Geometry: final body of the model. Coordinates: model frame, mm. A direction names the side the tool comes from. Coordinates: 2 decimals unless noted, no trailing zeros. Loops run counter-clockwise (first coordinate to the right, second up) from the corner with the lowest first, then second, coordinate; pieces in that order, holes last. Notation, with made-up numbers: (88.25, -18.5) -> (116.25, -18.5) arc R30 cw to (116.25, 12.5) -> close; hole circle Ø8 at (25.5, -28.75). An arc over 180 degrees is marked (long way). One line per item, written item: value. Start each with the question number.
Item 1: Mould query, pull axis Y, two halves, no side actions, for faces 4 (the flat face through (19.05, 13, -3)), 5 (the flat face through (20.5, 27, -2)), 6 (the cylindrical face through (9.27, 2.54, -14.83)). Classes: +Y half, -Y half, draft (parallel to the pull), parting line (faces both ways), or undercut.
Item 2: Section query A-A on z = -4. Return loops of the section in (x, y), then the cut area to 3 significant figures.
Item 3: Set-up query: faces 1 (the flat face through (12, 27, -1)), 2 (the flat face through (13, 15, -9.3)), 3 (the flat face through (5.7, 8.8, -4.8)). Return all of +Z, -Z, +X, -X, +Y, -Y with unobstructed straight access to the full face (end or side cutting, diameter ignored); none if empty.
Item 4: Ray query, probe 1 along Y at (x, z) = (23, -0.45); probe 2 along Y at (x, z) = (11, -1.5); probe 3 along Z at (x, y) = (18.75, 12). Return the intervals inside material, ascending. Write a range as from..to.
Item 5: Section query B-B on x = 15.5. Return loops of the section in (y, z).
Item 6: Contact query for flat-ended pins moving along their axis: pin 1 Ø5.5 at (x, y) = (9, 29) entering from +Z; pin 2 Ø12 at (x, y) = (14.5, 26) entering from -Z; pin 3 Ø1.1 at (y, z) = (13.5, -2.5) entering from +X; pin 4 Ø8 at (y, z) = (23.5, -7.5) entering from +X. Output: stop coordinate, or through.
Item 7: Section query C-C on y = 24.5. Return loops of the section in (x, z).
Item 8: Section query D-D on y = 8. Return loops of the section in (x, z), then the cut area to 3 significant figures.
from build123d import *

# Parameters (mm, degrees)
SKETCH_1_W             = 25
SKETCH_1_H             = 24
EXTRUDE_354_DEPTH      = 1
EXTRUDE_536_DEPTH      = 3.8
SKETCH_3_W             = 22
SKETCH_3_H             = 4.802295703
EXTRUDE_803_DEPTH      = 1.5
HOLE_WIZARD_953_D      = 0.5
HOLE_WIZARD_953_DEPTH  = 1
HOLE_WIZARD_1615_D     = 2
HOLE_WIZARD_1615_DEPTH = 16.4
SKETCH_12_W            = 16
SKETCH_12_H            = 1.5
EXTRUDE_2779_DEPTH     = 7.5


with BuildPart() as part:
    # Эскиз1 → Extrude 354 (new body)
    with BuildSketch(Plane(origin=(0, 0, -1), x_dir=(-1, 0, 0), z_dir=(0, 0, -1))):
        with Locations((-12.5, 12)):
            Rectangle(SKETCH_1_W, SKETCH_1_H)
    extrude(amount=-EXTRUDE_354_DEPTH)

    # Эскиз2 → Extrude 536 (add)
    with BuildSketch(Plane(origin=(0, 0, -1), x_dir=(-1, 0, 0), z_dir=(0, 0, -1))):
        with BuildLine():
            Line((-5.95, 10.75), (-3.949995117, 10.75))
            ThreePointArc((-3.949995117, 10.75), (-1.949995117, 8.75), (-3.949995117, 6.75))
            Line((-3.949995117, 6.75), (-5.95, 6.75))
            Line((-5.95, 6.75), (-5.95, 2.2))
            Line((-5.95, 2.2), (-19.05, 2.2))
            Line((-19.05, 2.2), (-19.05, 6.75))
            Line((-19.05, 6.75), (-21.050009766, 6.75))
            ThreePointArc((-21.050009766, 6.75), (-23.050009766, 8.75), (-21.050009766, 10.75))
            Line((-21.050009766, 10.75), (-19.05, 10.75))
            Line((-19.05, 10.75), (-19.05, 15.3))
            Line((-19.05, 15.3), (-5.95, 15.3))
            Line((-5.95, 15.3), (-5.95, 10.75))
        make_face()
    extrude(amount=EXTRUDE_536_DEPTH)

    # Эскиз3 → Extrude 803 (add)
    with BuildSketch(Plane(origin=(0, 0, -1), x_dir=(-1, 0, 0), z_dir=(0, 0, -1))):
        with Locations((-12.5, 21.098852149)):
            Rectangle(SKETCH_3_W, SKETCH_3_H)
    extrude(amount=EXTRUDE_803_DEPTH)

    # Эскиз4 → Revolve 894 (revolve)
    with BuildSketch(Plane.XZ.offset(-8.75), mode=Mode.PRIVATE) as revolve_894_sk:
        Polygon((19.1, -4.8), (12.5, -4.8), (12.5, -16.4), (19.5, -16.4), (19.5, -13.3), (18.25, -13.3), (18.25, -9.3), (19.1, -9.3), align=None)
    revolve(revolve_894_sk.sketch.rotate(Axis((12.5, 8.75, -4.8), (0, 0, -1)), 180), axis=Axis((12.5, 8.75, -4.8), (0, 0, -1)))

    # Hole Wizard 953
    with Locations(Plane.XY):
        with Locations((12.5, 8.75)):
            Hole(HOLE_WIZARD_953_D / 2, depth=HOLE_WIZARD_953_DEPTH)

    # Hole Wizard 1615
    with Locations(Plane.XY):
        with Locations((2, 2), (2, 15.5), (23, 15.5), (23, 2)):
            Hole(HOLE_WIZARD_1615_D / 2, depth=HOLE_WIZARD_1615_DEPTH)

    # Эскиз12 → Extrude 2779 (add)
    with BuildSketch(Plane(origin=(0, 23.5, 0), x_dir=(1, 0, 0), z_dir=(0, 1, 0))):
        with Locations((12.5, 1.75)):
            Rectangle(SKETCH_12_W, SKETCH_12_H)
    extrude(amount=EXTRUDE_2779_DEPTH)


solid = part.part
Reply:
1. face 4: undercut
1. face 5: draft
1. face 6: parting line
2. outline: (3.95, 6.75) -> (5.95, 6.75) -> (5.95, 2.2) -> (19.05, 2.2) -> (19.05, 6.75) -> (21.05, 6.75) arc R2 ccw to (21.05, 10.75) -> (19.05, 10.75) -> (19.05, 15.3) -> (5.95, 15.3) -> (5.95, 10.75) -> (3.95, 10.75) arc R2 ccw to start
2. area: 200 mm²
3. face 1: +Z, +X, -X, +Y
3. face 2: none
3. face 3: -X
4. probe 1: y = 0..1, 3..14.5, 16.5..24
4. probe 2: y = 2.2..15.3, 18.7..31
4. probe 3: z = -4.8..0
5. outline: (0, -1) -> (2.2, -1) -> (2.2, -4.8) -> (2.87, -4.8) -> (2.87, -9.3) -> (3.84, -9.3) -> (3.84, -13.3) -> (2.43, -13.3) -> (2.43, -16.4) -> (15.07, -16.4) -> (15.07, -13.3) -> (13.66, -13.3) -> (13.66, -9.3) -> (14.63, -9.3) -> (14.63, -4.8) -> (15.3, -4.8) -> (15.3, -1) -> (18.7, -1) -> (18.7, -2.5) -> (31, -2.5) -> (31, -1) -> (24, -1) -> (24, 0) -> (0, 0) -> close
6. pin 1: stops at z = -1
6. pin 2: stops at z = -2.5
6. pin 3: stops at x = 19.05
6. pin 4: passes through
7. outline: (4.5, -2.5) -> (20.5, -2.5) -> (20.5, -1) -> (4.5, -1) -> close
8. outline: (0, -1) -> (2.1, -1) -> (2.1, -4.8) -> (5.94, -4.8) -> (5.94, -9.3) -> (6.8, -9.3) -> (6.8, -13.3) -> (5.54, -13.3) -> (5.54, -16.4) -> (19.46, -16.4) -> (19.46, -13.3) -> (18.2, -13.3) -> (18.2, -9.3) -> (19.06, -9.3) -> (19.06, -4.8) -> (22.9, -4.8) -> (22.9, -1) -> (25, -1) -> (25, 0) -> (0, 0) -> close
8. area: 252 mm²
